```python
from build123d import *

# Parameters (mm, degrees)
SKETCH3_W           = 10
SKETCH3_H           = 5
BOSS_EXTRUDE1_DEPTH = 45
CHAMFER1_SIZE       = 1


with BuildPart() as part:
    # Sketch1 → Revolve1 (revolve)
    with BuildSketch(Plane.XY):
        Polygon((-136.678204549, 12.5), (-86.678204549, 12.5), (-86.678204549, 17), (-46.678204549, 17), (-46.678204549, 18), (-18.321795451, 23), (6.678204549, 23), (6.678204549, 17), (51.678204549, 17), (51.678204549, 14), (76.678204549, 14), (76.678204549, 12.5), (136.678204549, 12.5), (136.678204549, 0), (-136.678204549, 0), align=None)
    revolve(axis=Axis((136.678204549, 0, 0), (-1, 0, 0)))

    # Sketch3 → Boss-Extrude1 (add)
    with BuildSketch(Plane(origin=(51.678204549, 0, 0), x_dir=(0, 0, -1), z_dir=(1, 0, 0))):
        with Locations((0, 18.748076809)):
            Rectangle(SKETCH3_W, SKETCH3_H)
    extrude(amount=-BOSS_EXTRUDE1_DEPTH)

    # Chamfer1
    chamfer1_edges = [part.edges().sort_by_distance(p)[0] for p in [
        (136.678204549, -12.5, 0),
        (-136.678204549, -12.5, 0),
    ]]
    chamfer(chamfer1_edges, length=CHAMFER1_SIZE)


solid = part.part
```
Geometry check sheet. Reference: the model listing, model coordinates, mm. A direction names the side the tool comes from. Give positions to 0.01 mm unless a question says otherwise; leave off trailing zeros. Write each loop counter-clockwise with the first axis right and the second up, starting at its lowest first coordinate (ties: lowest second). Pieces come first, ordered by that corner, then holes. Notation, with made-up numbers: (63.25, 67.5) - (89.25, 67.5) arc R22 ccw to (89.25, 79.5) - close; hole circle Ø5 at (19.25, 39). An arc over 180 degrees is marked (long way). Use a Markdown table: item, result.
Q1. Section check D-D, the plane x = 105. Enter the section's corners in (y, z), then the cut area to 3 significant figures.
Computed:
| item | result |
|---|---|
| outline | circle Ø25 at (0, 0) |
| area | 491 mm² |
Q2. Go/stop test with flat-tipped pins: P1, Ø4, axis at x = 28.5, y = 19, coming from the +Z side; P2, Ø4, axis at x = 20, y = 19, coming from the -Z side; P3, Ø1.5, axis at y = -12.5, z = -18, coming from the +X side. Record where each tip stops, or that it passes through.
Computed:
| item | result |
|---|---|
| P1 | stops at z = 5 |
| P2 | stops at z = -5 |
| P3 | stops at x = 6.68 |
Q3. Set-up check for faces 1 (the face through (76.678, -5.3, -11.5)), 2 (the face through (29, 21.248, 0)), 3 (the face through (-66.398, 9.139, -14.334)): record each of +Z, -Z, +X, -X, +Y, -Y from which the full face is reachable in a straight line by a thin tool's end or side.
Computed:
| item | result |
|---|---|
| face 1 | +X |
| face 2 | +Z, -Z, +X, +Y |
| face 3 | -X |
Q4. Section check C-C, the plane x = 32.5. Enter the section's corners in (y, z).
Computed:
| item | result |
|---|---|
| outline | (16.25, -5) - (21.25, -5) - (21.25, 5) - (16.25, 5) arc R17 ccw (long way) to start |
Q5. Thickness scan on L1, parallel to X at y = -6, z = -14; L2, parallel to Z at x = -108.5, y = -1; L3, parallel to Z at x = 11.5, y = -1. Record the ranges inside material, lowest first. Write a range as [from, to].
Computed:
| item | result |
|---|---|
| L1 | x = [-86.68, 51.68] |
| L2 | z = [-12.46, 12.46] |
| L3 | z = [-16.97, 16.97] |
